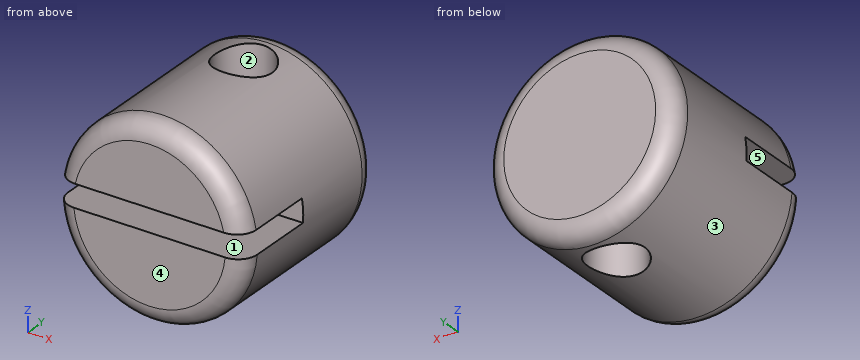
```python
from build123d import *

# Parameters (mm, degrees)
SKETCH1_R           = 12.7
BOSS_EXTRUDE1_DEPTH = 25.4
SKETCH2_R           = 3.81
CUT_EXTRUDE1_DEPTH  = 25.4
SKETCH3_W           = 3.048
SKETCH3_H           = 11.43
CUT_EXTRUDE2_DEPTH  = 25.4
FILLET1_R           = 2.54


with BuildPart() as part:
    # Sketch1 → Boss-Extrude1 (new body)
    with BuildSketch(Plane(origin=(0, 0, 0), x_dir=(1, 0, 0), z_dir=(0, 1, 0))):
        with Locations(Location((0, 0, 0), (0, 0, 270))):
            Circle(SKETCH1_R)
    extrude(amount=BOSS_EXTRUDE1_DEPTH)

    # Sketch2 → Cut-Extrude1 (cut, symmetric)
    with BuildSketch(Plane.XY):
        with Locations(Location((0, 18.286129729, 0), (0, 0, 90.000000018))):
            Circle(SKETCH2_R)
    extrude(amount=CUT_EXTRUDE1_DEPTH, both=True, mode=Mode.SUBTRACT)

    # Sketch3 → Cut-Extrude2 (cut, symmetric)
    with BuildSketch(Plane(origin=(0, 0, 0), x_dir=(0, 0, -1), z_dir=(1, 0, 0))):
        with Locations((-0.60404942, 5.715)):
            Rectangle(SKETCH3_W, SKETCH3_H)
    extrude(amount=CUT_EXTRUDE2_DEPTH, both=True, mode=Mode.SUBTRACT)

    # Fillet1
    fillet1_edges = [part.edges().sort_by_distance(p)[0] for p in [
        (0, 0, -12.7),
        (8.193405042, 0, 9.703510386),
        (0, 25.4, -12.7),
    ]]
    fillet(fillet1_edges, radius=FILLET1_R)


solid = part.part
```
Read the model definition and answer for the solid it produces. Units are mm, in the model's axes. Face numbers are marked on the shaded views. A direction names the side the tool comes from. Round coordinates to 2 decimals unless told otherwise and drop trailing zeros. Loops run counter-clockwise (first coordinate to the right, second up) from the corner with the lowest first, then second, coordinate; pieces in that order, holes last. Notation, with made-up numbers: (48.5, -10.5) -> (94.5, -10.5) arc R9 cw to (94.5, 6.5) -> close; hole circle Ø11 at (79, 49.5). An arc over 180 degrees is marked (long way). One line per item, written item: value.
1) Flat-ended cylindrical pins translate along their axes: P1, Ø3.5, axis at x = 2.5, y = 3.5, coming from the -Z side; P2, Ø4, axis at x = -5.5, z = -8, coming from the -Y side; P3, Ø1.5, axis at y = 9.5, z = 7, coming from the -X side; P4, Ø12, axis at y = 13, z = -7, coming from the +X side. Find the tip coordinate at first contact, or state that the pin passes through.
Answer list:
P1: stops at z = -12.68
P2: stops at y = 0
P3: stops at x = -11.06
P4: stops at x = 12.66
2) A cutting plane is placed at B-B (z = 0). Determine the outline of the cut face in (x, y).
Answer list:
outline: (-12.7, 11.43) -> (12.7, 11.43) -> (12.7, 22.86) arc R2.54 ccw to (10.16, 25.4) -> (-10.16, 25.4) arc R2.54 ccw to (-12.7, 22.86) -> close; hole circle Ø7.62 at (0, 18.29)
3) Consider L1, parallel to Y at x = 0, z = -2.25; L2, parallel to Z at x = -1.5, y = 10.5; L3, parallel to X at y = 19.5, z = -5. Determine where each line is inside the solid, lowest interval first. Write a range as [from, to].
Answer list:
L1: y = [0, 14.48], [22.1, 25.4]
L2: z = [-12.61, -0.92], [2.13, 12.61]
L3: x = [-11.67, -3.61], [3.61, 11.67]
4) For the marked faces 1 and 2, determine the directions among +Z, -Z, +X, -X, +Y, -Y from which every point of the face is accessible in a straight line to the end or side of a thin tool.
Answer list:
face 1: +X, -X, -Y
face 2: +Z, -Z
5) A cutting plane is placed at A-A (x = 0). Determine the outline of the cut face in (y, z).
Answer list:
outline: (0, -10.16) arc R2.54 ccw to (2.54, -12.7) -> (14.48, -12.7) -> (14.48, 12.7) -> (2.54, 12.7) arc R2.54 ccw to (0, 10.16) -> (0, 2.13) -> (11.43, 2.13) -> (11.43, -0.92) -> (0, -0.92) -> close; (22.1, -12.7) -> (22.86, -12.7) arc R2.54 ccw to (25.4, -10.16) -> (25.4, 10.16) arc R2.54 ccw to (22.86, 12.7) -> (22.1, 12.7) -> close
6) A cutting plane is placed at D-D (y = 17.5). Determine the outline of the cut face in (x, z).
Answer list:
outline: (-3.73, -12.14) -> (-3.73, 12.14) arc R12.7 ccw to start; (3.73, -12.14) arc R12.7 ccw to (3.73, 12.14) -> close
7) The mould has two halves that part along Z. Classify the marked faces 3, 4 and 5: pulls with the +Z half, pulls with the -Z half, needs draft (parallel to the pull), parting line crosses it, or undercut.
Answer list:
face 3: parting line crosses it
face 4: needs draft
face 5: undercut
8) A cutting plane is placed at C-C (y = 3.75). Determine the outline of the cut face in (x, z), and give its area (3 significant figures).
Answer list:
outline: (-12.67, -0.92) arc R12.7 ccw to (12.67, -0.92) -> close; (-12.52, 2.13) -> (12.52, 2.13) arc R12.7 ccw to start
area: 430 mm²
